Source: three-view drawing plus pictorial views. Frame: mm from the lowest corner of the part. Coordinates: 2 decimals unless noted, no trailing zeros. Order: outer loops, then holes, each group sorted by start corner. A loop starts at its lowest first (then second) coordinate and runs counter-clockwise, first axis right, second up. Notation, with made-up numbers: M 10.5,31 L 69.5,31 A30 cw 69.5,58 Z; hole C 12,-18.75 d3. An arc over 180 degrees is marked long. One line per question, with ' | ' between items.
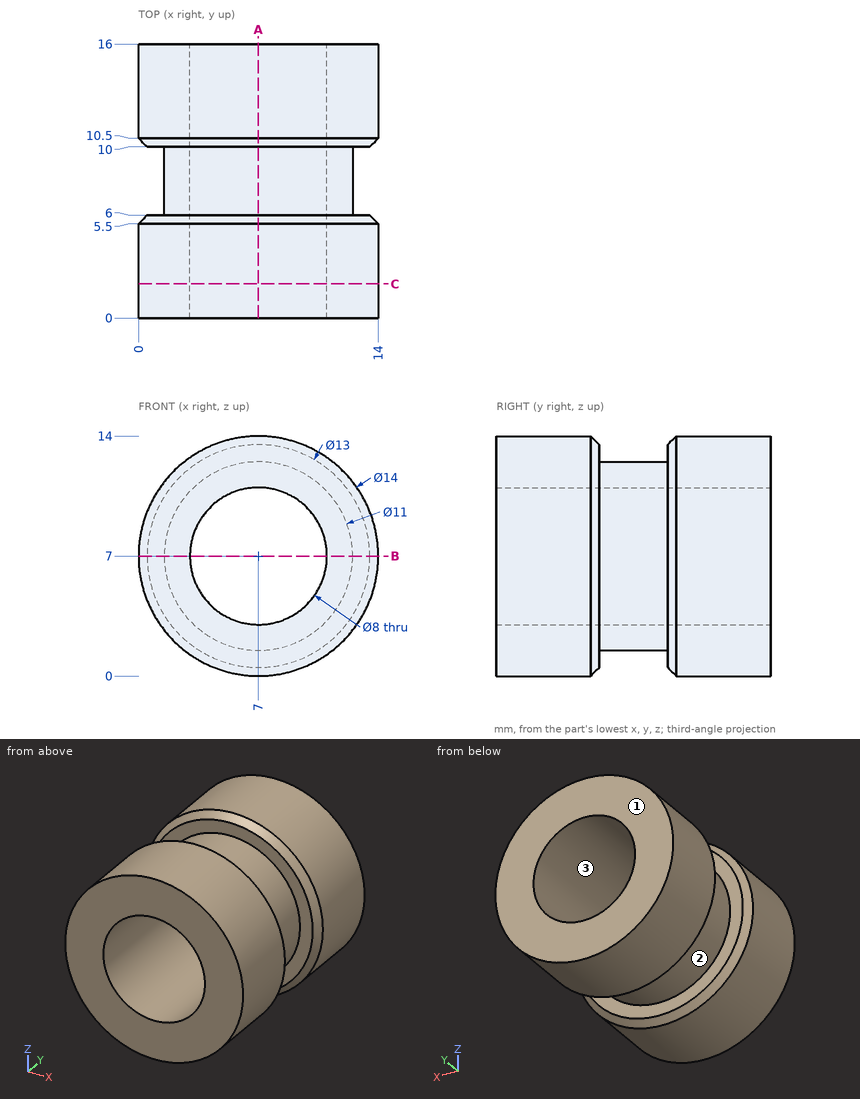
1. Material intervals for line 1 (Z direction, x = 7, y = 11.25); line 2 (Y direction, x = 11.5, z = 11); line 3 (Z direction, x = 7, y = 7.75), sorted ascending. Write a range as [from, to].
Response values:
line 1: z = [0, 3], [11, 14] | line 2: y = [0, 6], [10, 16] | line 3: z = [1.5, 3], [11, 12.5]
2. Section A-A, the plane x = 7. Output: boundary loops of the cut face in (y, z).
Response values:
outline: M 0,0 L 5.5,0 L 6,0.5 L 6,1.5 L 10,1.5 L 10,0.5 L 10.5,0 L 16,0 L 16,3 L 0,3 Z; M 0,11 L 16,11 L 16,14 L 10.5,14 L 10,13.5 L 10,12.5 L 6,12.5 L 6,13.5 L 5.5,14 L 0,14 Z
3. Draft query along X for the marked faces 1, 2 and 3. Return one class per face: pulls with the +X half, pulls with the -X half, needs draft (parallel to the pull), parting line crosses it, or undercut.
Response values:
face 1: needs draft | face 2: parting line crosses it | face 3: undercut
4. Pin query (flat end, axial travel): P1, Ø1, axis at x = 2.5, y = 14.5, coming from the +Z side; P2, Ø8, axis at x = 12.5, y = 4.5, coming from the -Z side; P3, Ø5, axis at x = 10.5, y = 9.5, coming from the +Z side. Return the tip coordinate at first contact, or that it passes through.
Response values:
P1: stops at z = 12.74 | P2: stops at z = 0.16 | P3: stops at z = 13.89
5. Section C-C, the plane y = 2. Output: boundary loops of the cut face in (x, z).
Response values:
outline: C 7,7 d14; hole C 7,7 d8
6. Section B-B, the plane z = 7. Output: boundary loops of the cut face in (x, y), and give its area (3 significant figures).
Response values:
outline: M 0,0 L 3,0 L 3,16 L 0,16 L 0,10.5 L 0.5,10 L 1.5,10 L 1.5,6 L 0.5,6 L 0,5.5 Z; M 11,0 L 14,0 L 14,5.5 L 13.5,6 L 12.5,6 L 12.5,10 L 13.5,10 L 14,10.5 L 14,16 L 11,16 Z | area: 83.5 mm^2
